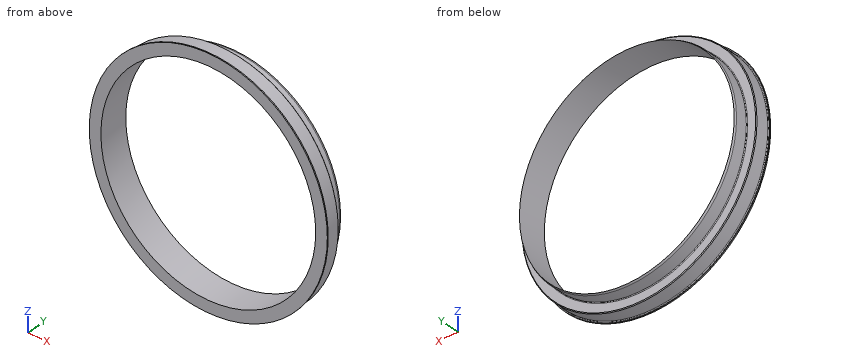
from build123d import *

# Parameters (mm, degrees)
FILLET1_R     = 0.508
CHAMFER1_SIZE = 0.508


with BuildPart() as part:
    # Sketch1 → Revolve1 (revolve)
    with BuildSketch(Plane.XY):
        Polygon((76.2, 21.082), (76.2, 0), (84.455, 0), (84.455, 0.762), (83.439, 0.762), (83.439, 10.922), (76.708, 10.922), (76.708, 19.686281471), align=None)
    revolve(axis=Axis((0, 28.738956579, 0), (0, -1, 0)))

    # Fillet1
    fillet1_edges = [part.edges().sort_by_distance(p)[0] for p in [
        (-83.439, 0.762, 0),
        (-76.708, 10.922, 0),
    ]]
    fillet(fillet1_edges, radius=FILLET1_R)

    # Chamfer1
    chamfer1_edges = [part.edges().sort_by_distance(p)[0] for p in [
        (-83.439, 10.922, 0),
    ]]
    chamfer(chamfer1_edges, length=CHAMFER1_SIZE)


solid = part.part
The model under review builds one solid part; all positions refer to its coordinate system, in mm. Round coordinates to 2 decimals unless told otherwise and drop trailing zeros. Loops run counter-clockwise (first coordinate to the right, second up) from the corner with the lowest first, then second, coordinate; pieces in that order, holes last. Notation, with made-up numbers: M 1,20.5 L 59,20.5 A32 cw 59,53.5 Z; hole C -33.5,19.25 d9. An arc over 180 degrees is marked long. Answer as a JSON object with one key per item and string values.
Item 1: For line 1 along Z through (x, y) = (0, 13.25); line 2 along Z through (x, y) = (0, 5.5); line 3 along X through (y, z) = (3.5, 58), list the stretches that pass through material, from the lowest coordinate up.
Check sheet entries:
{"line 1": "-76.71 to -76.2, 76.2 to 76.71", "line 2": "-83.44 to -76.2, 76.2 to 83.44", "line 3": "-59.98 to -49.42, 49.42 to 59.98"}
Item 2: We need section B-B, the plane x = 0. State the section outline as (y, z) points (3 decimals).
Check sheet entries:
{"outline": "M 0,-84.455 L 0.762,-84.455 L 0.762,-83.947 A0.508 cw 1.27,-83.439 L 10.414,-83.439 L 10.922,-82.931 L 10.922,-77.216 A0.508 cw 11.43,-76.708 L 19.686,-76.708 L 21.082,-76.2 L 0,-76.2 Z; M 0,76.2 L 21.082,76.2 L 19.686,76.708 L 11.43,76.708 A0.508 cw 10.922,77.216 L 10.922,82.931 L 10.414,83.439 L 1.27,83.439 A0.508 cw 0.762,83.947 L 0.762,84.455 L 0,84.455 Z"}
Item 3: Clearance check with flat-ended pins moving along their axes: P1, Ø12, axis at y = 17, z = 43, coming from the -X side; P2, Ø5, axis at y = 18, z = 53, coming from the -X side; P3, Ø6, axis at y = 3.5, z = -60, coming from the +X side. State where each tip first meets the part, or that it passes through.
Check sheet entries:
{"P1": "x = -67.19", "P2": "x = -57.74", "P3": "x = 60.93"}
Item 4: We need section A-A, the plane z = 0. State the section outline as (x, y) points (3 decimals), and give its area (3 significant figures).
Check sheet entries:
{"outline": "M -84.455,0 L -76.2,0 L -76.2,21.082 L -76.708,19.686 L -76.708,11.43 A0.508 cw -77.216,10.922 L -82.931,10.922 L -83.439,10.414 L -83.439,1.27 A0.508 cw -83.947,0.762 L -84.455,0.762 Z; M 76.2,0 L 84.455,0 L 84.455,0.762 L 83.947,0.762 A0.508 cw 83.439,1.27 L 83.439,10.414 L 82.931,10.922 L 77.216,10.922 A0.508 cw 76.708,11.43 L 76.708,19.686 L 76.2,21.082 Z", "area": "169 mm2"}
